Here's how the part is built. I have some questions about the finished solid (model axes, mm). A direction names the side the tool comes from. Round coordinates to 2 decimals unless told otherwise and drop trailing zeros. Order: outer loops, then holes, each group sorted by start corner. A loop starts at its lowest first (then second) coordinate and runs counter-clockwise, first axis right, second up.
```python
from build123d import *


with BuildPart() as part:
    # Sketch1 → Revolve-Thin1 (revolve)
    with BuildSketch(Plane.XY):
        with BuildLine():
            Line((0, 0), (-75, 0))
            ThreePointArc((-75, 0), (-81.436643777, 29.696137594), (-83.665296811, 60))
            ThreePointArc((-83.665296811, 60), (-96.158654713, 165.616239893), (-10, 227.96654333))
            Line((-10, 227.96654333), (-10, 277.96654333))
            Line((-10, 277.96654333), (-9, 277.96654333))
            Line((-9, 277.96654333), (-9, 227.053663621))
            ThreePointArc((-9, 227.053663621), (-95.127140134, 165.477462314), (-82.666179465, 60.338329285))
            ThreePointArc((-82.666179465, 60.338329285), (-80.523769647, 30.37601117), (-74.248389625, 1))
            Line((-74.248389625, 1), (0, 1))
            Line((0, 1), (0, 0))
        make_face()
    revolve(axis=Axis((0, 0, 0), (0, 1, 0)))


solid = part.part
```
1. If we mould it in two halves opening along X, with no side actions, what happens to faces 3 (the flat face through (9, 277.967, 2)), 4 (the cylindrical face through (2.17, 253.32, -9.76)), 5 (the cylindrical face through (1.172, 252.154, 8.923))? For each: released by +X, released by -X, zero draft, split by the parting line, or undercut.
Evaluation:
face 3: zero draft
face 4: split by the parting line
face 5: undercut
2. I need wall thicknesses on probe 1 along Z at (x, y) = (0, 261); probe 2 along X at (y, z) = (252, 1); probe 3 along X at (y, z) = (131, 92.5). Which ranges of each line are inside material? Lowest first, please.
Evaluation:
probe 1: z = -10 to -9, 9 to 10
probe 2: x = -9.95 to -8.94, 8.94 to 9.95
probe 3: x = -49.11 to -46.93, 46.93 to 49.11
3. If we section it at B-B, the plane z = -89: Write out the boundary of the cut face in (x, y), and give its area (3 significant figures).
Evaluation:
outline: circle Ø111.43 at (0, 123.44); hole circle Ø107.61 at (0, 123.44)
area: 657 mm2
4. On a 3-axis mill with a long thin cutter (end or side, diameter ignored), from which of +Z, -Z, +X, -X, +Y, -Y can I reach the whole of each face in a straight line? I mean faces 1 (the flat face through (1, 1, 1)), 2 (the flat face through (-1, 0, 1)). Say none if no direction works.
Evaluation:
face 1: none
face 2: +Z, -Z, +X, -X, -Y
5. I'm going to push flat-ended pins straight in: P1, Ø4, axis at y = 89, z = -66.5, coming from the +X side; P2, Ø5, axis at x = -34, y = 103.5, coming from the -Z side; P3, Ø10, axis at y = 180.5, z = 51, coming from the +X side. Where does each tip first touch, or does it pass through?
Evaluation:
P1: stops at x = 75.58
P2: stops at z = -98.3
P3: stops at x = 76.87
6. If we section it at A-A, the plane y = 248.5: Write out the boundary of the cut face in (x, z).
Evaluation:
outline: circle Ø20 at (0, 0); hole circle Ø18 at (0, 0)
